Could you check a few things on this model? Use its own coordinates, in mm. Face numbers are marked on the shaded views. A direction names the side the tool comes from. Coordinates: 2 decimals unless noted, no trailing zeros. Write each loop counter-clockwise with the first axis right and the second up, starting at its lowest first coordinate (ties: lowest second). Pieces come first, ordered by that corner, then holes. Notation, with made-up numbers: M -21,63.5 L 8,63.5 A22 cw 8,83.5 Z; hole C 8,-31 d6. An arc over 180 degrees is marked long. Answer as CSV lines item,"result". Start each with the question number.
Item 1: We'd pull the mould along X, two halves only. Please class the marked faces 1, 2 and 3: +X half, -X half, draft (parallel to the pull), parting line (faces both ways), or undercut.
Item 2: Suppose I cut it at A-A, the plane z = 3. State how many separate pieces and enclosed holes the cut face has, and give its area (3 significant figures).
Item 3: Suppose I cut it at B-B, the plane y = 14.76. Write out the boundary of the cut face in (x, z) (3 decimals), and give its area (3 significant figures).
Item 4: Suppose I cut it at C-C, the plane y = -13.49. Write out the boundary of the cut face in (x, z).
Item 5: Suppose I cut it at D-D, the plane z = 9.5. Write out the boundary of the cut face in (x, y).
Item 6: On a 3-axis mill with a long thin cutter (end or side, diameter ignored), from which of +Z, -Z, +X, -X, +Y, -Y can I reach the whole of each face in a straight line? I mean the marked faces 4 and 5. Say none if no direction works.
Item 7: If I drill on line 1 along Y through (x, z) = (48.25, 14.74) (3 decimals); line 2 along Y through (x, z) = (-11, 11.5); line 3 along X through (y, z) = (-22.5, 19.25), over which ranges is the centre line in solid material (lowest first)? Write a range as [from, to].
Item 8: I'm going to push flat-ended pins straight in: P1, Ø4.5, axis at y = -13.49, z = 14.74, coming from the +X side; P2, Ø1.5, axis at x = -20, y = 3, coming from the +Z side; P3, Ø3, axis at y = 14.76, z = 14.74, coming from the +X side; P4, Ø2.5, axis at x = 44.5, y = 24.5, coming from the +Z side. Where does each tip first touch, or does it pass through?
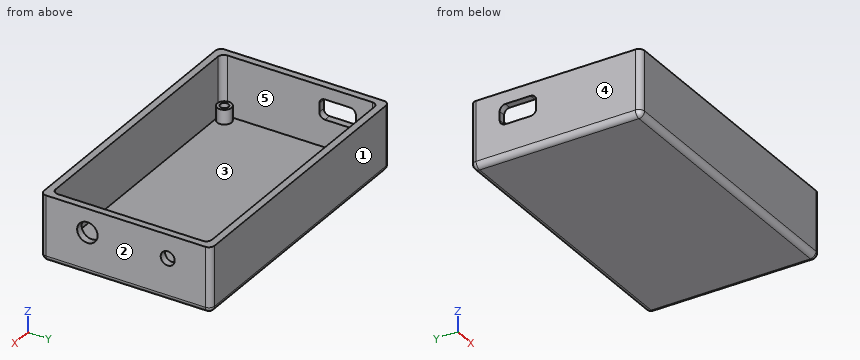
```python
from build123d import *

# Parameters (mm, degrees)
SKETCH1_W                 = 100
SKETCH1_H                 = 60
BOSS_EXTRUDE1_DEPTH       = 23
SKETCH2_W                 = 95
SKETCH2_H                 = 55
CUT_EXTRUDE1_DEPTH        = 21
SKETCH3_R                 = 2.51
SKETCH3_R_2               = 1.5
BOSS_EXTRUDE6_DEPTH       = 5.112
MIRROR2_COPY_1_SKETCH_R   = 2.51
MIRROR2_COPY_1_SKETCH_R_2 = 1.5
MIRROR2_COPY_1_DEPTH      = 5.112
FILLET1_R                 = 2
CUT_EXTRUDE2_REACH        = 108.907
SKETCH4_W                 = 7.027664142
SKETCH4_H                 = 12.863273411
FILLET2_R                 = 2
CUT_EXTRUDE3_REACH        = 108.907
SKETCH5_R                 = 3.6
SKETCH5_R_2               = 2.475


with BuildPart() as part:
    # Sketch1 → Boss-Extrude1 (new body)
    with BuildSketch(Plane.XY):
        Rectangle(SKETCH1_W, SKETCH1_H)
    extrude(amount=BOSS_EXTRUDE1_DEPTH)

    # Sketch2 → Cut-Extrude1 (cut)
    with BuildSketch(Plane.XY.offset(23)):
        Rectangle(SKETCH2_W, SKETCH2_H)
    extrude(amount=-CUT_EXTRUDE1_DEPTH, mode=Mode.SUBTRACT)

    # Sketch3 → Boss-Extrude6 (add)
    with BuildSketch(Plane.XY.offset(2)):
        with Locations((-44.89, 24.89)):
            Circle(SKETCH3_R)
        with Locations((-44.89, 24.89)):
            Circle(SKETCH3_R_2, mode=Mode.SUBTRACT)
    boss_extrude6 = extrude(amount=BOSS_EXTRUDE6_DEPTH)

    # Mirror1: Boss-Extrude6 across plane
    add(boss_extrude6.mirror(Plane.ZX))

    # Mirror2: Boss-Extrude6 across plane
    add(boss_extrude6.mirror(Plane(origin=(0, 0, 0), x_dir=(0, 0, 1), z_dir=(1, 0, 0))))

    # Mirror2 copy 1 sketch → Mirror2 copy 1 (add)
    with BuildSketch(Plane(origin=(0, 0, 2), x_dir=(-1, 0, 0), z_dir=(0, 0, 1))):
        with Locations((-44.89, 24.89)):
            Circle(MIRROR2_COPY_1_SKETCH_R)
        with Locations((-44.89, 24.89)):
            Circle(MIRROR2_COPY_1_SKETCH_R_2, mode=Mode.SUBTRACT)
    extrude(amount=MIRROR2_COPY_1_DEPTH)

    # Fillet1
    fillet1_edges = [part.edges().sort_by_distance(p)[0] for p in [
        (-47.5, 27.5, 12.5),
        (47.5, 27.5, 12.5),
        (47.5, -27.5, 12.5),
        (-47.5, -27.5, 12.5),
        (0, -30, 0),
        (-50, 0, 0),
        (0, 30, 0),
        (50, 0, 0),
        (50, -30, 11.5),
        (-50, -30, 11.5),
        (-50, 30, 11.5),
        (50, 30, 11.5),
    ]]
    fillet(fillet1_edges, radius=FILLET1_R)

    # Sketch4 → Cut-Extrude2 (cut, up to next)
    with BuildSketch(Plane.ZY.offset(50), mode=Mode.PRIVATE) as cut_extrude2_sk1:
        with Locations((15.125832071, 13.291636706)):
            Rectangle(SKETCH4_W, SKETCH4_H)
    cut_extrude2_tool1 = extrude(cut_extrude2_sk1.sketch, amount=-CUT_EXTRUDE2_REACH, mode=Mode.PRIVATE) & part.part
    add(cut_extrude2_tool1.solids().sort_by_distance((-50, 13.291637, 15.125832))[0], mode=Mode.SUBTRACT)

    # Fillet2
    fillet2_edges = [part.edges().sort_by_distance(p)[0] for p in [
        (-48.75, 19.723273411, 11.612),
        (-48.75, 6.86, 11.612),
        (-48.75, 6.86, 18.639664142),
        (-48.75, 19.723273411, 18.639664142),
    ]]
    fillet(fillet2_edges, radius=FILLET2_R)

    # Sketch5 → Cut-Extrude3 (cut, up to next)
    with BuildSketch(Plane(origin=(50, 0, 0), x_dir=(0, 0, -1), z_dir=(1, 0, 0)), mode=Mode.PRIVATE) as cut_extrude3_sk1:
        with Locations((-14.74, -13.49)):
            Circle(SKETCH5_R)
    cut_extrude3_tool1 = extrude(cut_extrude3_sk1.sketch, amount=-CUT_EXTRUDE3_REACH, mode=Mode.PRIVATE) & part.part
    # Sketch5 → Cut-Extrude3 (cut, up to next)
    with BuildSketch(Plane(origin=(50, 0, 0), x_dir=(0, 0, -1), z_dir=(1, 0, 0)), mode=Mode.PRIVATE) as cut_extrude3_sk2:
        with Locations((-14.74, 14.76)):
            Circle(SKETCH5_R_2)
    cut_extrude3_tool2 = extrude(cut_extrude3_sk2.sketch, amount=-CUT_EXTRUDE3_REACH, mode=Mode.PRIVATE) & part.part
    add(cut_extrude3_tool1.solids().sort_by_distance((50, -13.49, 14.74))[0], mode=Mode.SUBTRACT)
    add(cut_extrude3_tool2.solids().sort_by_distance((50, 14.76, 14.74))[0], mode=Mode.SUBTRACT)


solid = part.part
```
Ans:
1,face 1,"draft"
1,face 2,"+X half"
1,face 3,"undercut"
2,separate pieces,"5"
2,enclosed holes,"5"
2,area,"826 mm^2"
3,outline,"M -50,2 A2 ccw -48,0 L 48,0 A2 ccw 50,2 L 50,12.265 L 47.5,12.265 L 47.5,2 L -47.5,2 L -47.5,11.612 L -50,11.612 Z; M -50,18.64 L -47.5,18.64 L -47.5,23 L -50,23 Z; M 47.5,17.215 L 50,17.215 L 50,23 L 47.5,23 Z"
3,area,"273 mm^2"
4,outline,"M -50,2 A2 ccw -48,0 L 48,0 A2 ccw 50,2 L 50,11.14 L 47.5,11.14 L 47.5,2 L -47.5,2 L -47.5,23 L -50,23 Z; M 47.5,18.34 L 50,18.34 L 50,23 L 47.5,23 Z"
5,outline,"M -50,-28 A2 ccw -48,-30 L 48,-30 A2 ccw 50,-28 L 50,28 A2 ccw 48,30 L -48,30 A2 ccw -50,28 Z; hole M -47.5,-25.5 A2 ccw -45.5,-27.5 L 45.5,-27.5 A2 ccw 47.5,-25.5 L 47.5,25.5 A2 ccw 45.5,27.5 L -45.5,27.5 A2 ccw -47.5,25.5 Z"
6,face 4,"+Z, -Z, -X, +Y, -Y"
6,face 5,"+Z"
7,line 1,"y = [-29.984, -17.09], [-9.89, 12.285], [17.235, 29.984]"
7,line 2,"y = [-30, -27.5], [27.5, 30]"
7,line 3,"x = [-50, -47.5], [47.5, 50]"
8,P1,"stops at x = -47.5"
8,P2,"stops at z = 2"
8,P3,"passes through"
8,P4,"stops at z = 7.11"
